from build123d import *

# Parameters (mm, degrees)
SKETCH_1_R          = 1.6
EXTRUDE_1_DEPTH     = 7
SKETCH_2_W          = 90
SKETCH_2_H          = 120
SKETCH_2_W_2        = 80
SKETCH_2_H_2        = 110
EXTRUDE_2_DEPTH     = 60
SKETCH_3_W          = 56
SKETCH_3_H          = 36
SKETCH_3_W_2        = 50
SKETCH_3_H_2        = 30
EXTRUDE_3_DEPTH     = 10
SKETCH_5_W          = 56
SKETCH_5_H          = 3
EXTRUDE_4_DEPTH     = 20
SKETCH_6_W          = 30
SKETCH_6_H          = 5
EXTRUDE_5_DEPTH     = 60
CUT_EXTRUDE_1_DEPTH = 10
EXTRUDE_6_DEPTH     = 5
CUT_EXTRUDE_2_DEPTH = 10
CUT_EXTRUDE_3_DEPTH = 10
CUT_EXTRUDE_4_DEPTH = 10


with BuildPart() as part:
    # 草图1 → 凸台-拉伸1 (new body)
    with BuildSketch(Plane(origin=(0, 0, 0), x_dir=(1, 0, 0), z_dir=(0, 1, 0))):
        with BuildLine():
            Line((-85.25974026, 139.090909091), (74.74025974, 139.090909091))
            ThreePointArc((74.74025974, 139.090909091), (81.811327552, 136.161976903), (84.74025974, 129.090909091))
            Line((84.74025974, 129.090909091), (84.74025974, -70.909090909))
            ThreePointArc((84.74025974, -70.909090909), (81.811327552, -77.980158721), (74.74025974, -80.909090909))
            Line((74.74025974, -80.909090909), (-85.25974026, -80.909090909))
            ThreePointArc((-85.25974026, -80.909090909), (-92.330808072, -77.980158721), (-95.25974026, -70.909090909))
            Line((-95.25974026, -70.909090909), (-95.25974026, 129.090909091))
            ThreePointArc((-95.25974026, 129.090909091), (-92.330808072, 136.161976903), (-85.25974026, 139.090909091))
        make_face()
        with Locations((-62.25974026, 89.090909091)):
            Circle(SKETCH_1_R, mode=Mode.SUBTRACT)
        with Locations((51.74025974, 89.090909091)):
            Circle(SKETCH_1_R, mode=Mode.SUBTRACT)
        with Locations((-62.25974026, -30.909090909)):
            Circle(SKETCH_1_R, mode=Mode.SUBTRACT)
        with Locations((51.74025974, -30.909090909)):
            Circle(SKETCH_1_R, mode=Mode.SUBTRACT)
    extrude(amount=EXTRUDE_1_DEPTH)

    # 草图2 → 凸台-拉伸2 (add)
    with BuildSketch(Plane.XZ):
        with Locations((-5.25974026, -64.090909091)):
            Rectangle(SKETCH_2_W, SKETCH_2_H)
        with Locations((-5.25974026, -64.090909091)):
            Rectangle(SKETCH_2_W_2, SKETCH_2_H_2, mode=Mode.SUBTRACT)
    extrude(amount=EXTRUDE_2_DEPTH)

    # 草图3 → 凸台-拉伸3 (add)
    with BuildSketch(Plane.XZ):
        with Locations((-5.25974026, 22.137368895)):
            Rectangle(SKETCH_3_W, SKETCH_3_H)
        with Locations((-5.25974026, 22.137368895)):
            Rectangle(SKETCH_3_W_2, SKETCH_3_H_2, mode=Mode.SUBTRACT)
    extrude(amount=EXTRUDE_3_DEPTH)

    # 草图5 → 凸台-拉伸4 (add)
    with BuildSketch(Plane.XZ.offset(10)):
        with Locations((-5.25974026, 5.637368895)):
            Rectangle(SKETCH_5_W, SKETCH_5_H)
    extrude(amount=EXTRUDE_4_DEPTH)

    # 草图6 → 凸台-拉伸5 (add)
    with BuildSketch(Plane.XZ):
        with Locations((-5.25974026, 69.33277689)):
            Rectangle(SKETCH_6_W, SKETCH_6_H)
    extrude(amount=EXTRUDE_5_DEPTH)

    # 草图8 → 切除-拉伸1 (cut)
    with BuildSketch(Plane.XY.offset(71.83277689)):
        with BuildLine():
            Line((-6.25974026, -43), (-10.25974026, -60))
            Line((-10.25974026, -60), (-0.25974026, -60))
            Line((-0.25974026, -60), (-4.25974026, -43))
            ThreePointArc((-4.25974026, -43), (-4.523672282, -41.881966011), (-5.25974026, -41))
            ThreePointArc((-5.25974026, -41), (-5.995808237, -41.881966011), (-6.25974026, -43))
        make_face()
    extrude(amount=-CUT_EXTRUDE_1_DEPTH, mode=Mode.SUBTRACT)

    # 草图9 → 凸台-拉伸6 (add)
    with BuildSketch(Plane.XY.offset(71.83277689)):
        Polygon((-6.25974026, -60), (-9.789152024, -58), (-10.25974026, -60), align=None)
        Polygon((-4.25974026, -60), (-0.25974026, -60), (-0.730328495, -58), align=None)
    extrude(amount=-EXTRUDE_6_DEPTH)

    # 草图10 → 切除-拉伸2 (cut)
    with BuildSketch(Plane.XZ):
        with BuildLine():
            Line((-64.659020205, -16.259764427), (-64.659020205, -61.488758584))
            ThreePointArc((-64.659020205, -61.488758584), (-73.36978945, -70.199527829), (-82.080558695, -61.488758584))
            Line((-82.080558695, -61.488758584), (-82.080558695, -16.259764427))
            ThreePointArc((-82.080558695, -16.259764427), (-73.36978945, -7.548995182), (-64.659020205, -16.259764427))
        make_face()
        with BuildLine():
            Line((67.459227113, -16.259764427), (67.459227113, -61.488758584))
            ThreePointArc((67.459227113, -61.488758584), (57.906863547, -71.04112215), (48.354499981, -61.488758584))
            Line((48.354499981, -61.488758584), (48.354499981, -16.259764427))
            ThreePointArc((48.354499981, -16.259764427), (57.906863547, -6.707400861), (67.459227113, -16.259764427))
        make_face()
    extrude(amount=-CUT_EXTRUDE_2_DEPTH, mode=Mode.SUBTRACT)

    # 草图11 → 切除-拉伸3 (cut)
    with BuildSketch(Plane.XZ):
        with BuildLine():
            Line((-80.892767317, 71.523985845), (-45.044601578, 71.523985845))
            ThreePointArc((-45.044601578, 71.523985845), (-38.176495058, 64.655879325), (-45.044601578, 57.787772805))
            Line((-45.044601578, 57.787772805), (-80.892767317, 57.787772805))
            ThreePointArc((-80.892767317, 57.787772805), (-87.760873837, 64.655879325), (-80.892767317, 71.523985845))
        make_face()
        with BuildLine():
            Line((39.550368976, 72.361559811), (65.180132332, 72.361559811))
            ThreePointArc((65.180132332, 72.361559811), (72.885812818, 64.655879325), (65.180132332, 56.950198839))
            Line((65.180132332, 56.950198839), (39.550368976, 56.950198839))
            ThreePointArc((39.550368976, 56.950198839), (31.84468849, 64.655879325), (39.550368976, 72.361559811))
        make_face()
    extrude(amount=-CUT_EXTRUDE_3_DEPTH, mode=Mode.SUBTRACT)

    # 草图12 → 切除-拉伸4 (cut)
    with BuildSketch(Plane.XZ):
        with BuildLine():
            Line((-65.903935016, -99.695986078), (-65.903935016, -125.770060152))
            ThreePointArc((-65.903935016, -125.770060152), (-72.642178878, -132.508304014), (-79.38042274, -125.770060152))
            Line((-79.38042274, -125.770060152), (-79.38042274, -99.695986078))
            ThreePointArc((-79.38042274, -99.695986078), (-72.642178878, -92.957742216), (-65.903935016, -99.695986078))
        make_face()
        with BuildLine():
            Line((66.517205225, -99.695986078), (66.517205225, -125.770060152))
            ThreePointArc((66.517205225, -125.770060152), (61.243796985, -131.043468392), (55.970388746, -125.770060152))
            Line((55.970388746, -125.770060152), (55.970388746, -99.695986078))
            ThreePointArc((55.970388746, -99.695986078), (61.243796985, -94.422577838), (66.517205225, -99.695986078))
        make_face()
    extrude(amount=-CUT_EXTRUDE_4_DEPTH, mode=Mode.SUBTRACT)


solid = part.part
Work out the finished part from the listing and answer in its coordinate system (mm). A direction names the side the tool comes from. Give positions to 0.01 mm unless a question says otherwise; leave off trailing zeros. Order: outer loops, then holes, each group sorted by start corner. A loop starts at its lowest first (then second) coordinate and runs counter-clockwise, first axis right, second up. Notation, with made-up numbers: (-7, 79.25) -> (32, 79.25) arc R28 cw to (32, 117.25) -> close; hole circle Ø8 at (44.5, 78.5). An arc over 180 degrees is marked (long way). Answer as a JSON object with one key per item and string values. Group by question number.
1. Section D-D on x = -14 is taken. Determine the outline of the cut face in (y, z), plus the area to 3 significant figures.
2. Section C-C on z = -49 is taken. Determine the outline of the cut face in (x, y).
3. Section B-B on y = -36 is taken. Determine the outline of the cut face in (x, z), plus the area to 3 significant figures.
4. A tool of negligible diameter and unlimited length cuts with its end or side. For faces 1 (the flat face through (-5, 0, 22)), 2 (the flat face through (-5, -30, 71.833)), 3 (the flat face through (-63, 3, 71.524)), from which of +Z, -Z, +X, -X, +Y, -Y can it reach the whole face along a straight path? Write none if from no direction.
5. Flat-ended cylindrical pins translate along their axes: pin 1 Ø18 at (x, y) = (-9.5, -28.5) entering from -Z; pin 2 Ø8 at (y, z) = (-5.5, 20) entering from +X; pin 3 Ø2 at (y, z) = (-37.5, -63) entering from +X. Find the tip coordinate at first contact, or state that the pin passes through.
6. The mould has two halves that part along X. Classify faces 4 (the cylindrical face through (-72.494, 3.451, -132.507)), 5 (the flat face through (39.74, -30, -65)), 6 (the flat face through (-5, -30, 66.833)), 7 (the flat face through (-95.26, 3, -28)): released by +X, released by -X, zero draft, split by the parting line, or undercut.
7. Section A-A on y = -23 is taken. Determine the outline of the cut face in (x, z).
8. Consider line 1 along Z through (x, y) = (-30.5, -14); line 2 along X through (y, z) = (-53, -20); line 3 along Z through (x, y) = (14.5, -3). Determine where each line is inside the solid, lowest interval first. Write a range as [from, to].
Result sheet:
{
 "1": {"outline": "(-60, -124.09) -> (0, -124.09) -> (0, -139.09) -> (7, -139.09) -> (7, 80.91) -> (0, 80.91) -> (0, 71.83) -> (-60, 71.83) -> (-60, 66.83) -> (0, 66.83) -> (0, 40.14) -> (-10, 40.14) -> (-10, 37.14) -> (0, 37.14) -> (0, 7.14) -> (-30, 7.14) -> (-30, 4.14) -> (0, 4.14) -> (0, -4.09) -> (-60, -4.09) -> (-60, -9.09) -> (0, -9.09) -> (0, -119.09) -> (-60, -119.09) -> close", "area": "2,560 mm^2"},
 "2": {"outline": "(-95.26, 0) -> (-82.08, 0) -> (-82.08, 7) -> (-95.26, 7) -> close; (-64.66, 0) -> (-50.26, 0) -> (-50.26, -60) -> (-45.26, -60) -> (-45.26, 0) -> (34.74, 0) -> (34.74, -60) -> (39.74, -60) -> (39.74, 0) -> (48.35, 0) -> (48.35, 7) -> (-64.66, 7) -> close; (67.46, 0) -> (84.74, 0) -> (84.74, 7) -> (67.46, 7) -> close"},
 "3": {"outline": "(-50.26, -124.09) -> (39.74, -124.09) -> (39.74, -4.09) -> (-50.26, -4.09) -> close; (-20.26, 66.83) -> (9.74, 66.83) -> (9.74, 71.83) -> (-20.26, 71.83) -> close; hole (-45.26, -119.09) -> (34.74, -119.09) -> (34.74, -9.09) -> (-45.26, -9.09) -> close", "area": "2,150 mm^2"},
 "4": {"face 1": "-Y", "face 2": "+Z, +X, -X, -Y", "face 3": "+Y, -Y"},
 "5": {"pin 1": "stops at z = -124.09", "pin 2": "stops at x = 22.74", "pin 3": "stops at x = 39.74"},
 "6": {"face 4": "undercut", "face 5": "released by +X", "face 6": "zero draft", "face 7": "released by -X"},
 "7": {"outline": "(-50.26, -124.09) -> (39.74, -124.09) -> (39.74, -4.09) -> (-50.26, -4.09) -> close; (-33.26, 4.14) -> (22.74, 4.14) -> (22.74, 7.14) -> (-33.26, 7.14) -> close; (-20.26, 66.83) -> (9.74, 66.83) -> (9.74, 71.83) -> (-20.26, 71.83) -> close; hole (-45.26, -119.09) -> (34.74, -119.09) -> (34.74, -9.09) -> (-45.26, -9.09) -> close"},
 "8": {"line 1": "z = [-124.09, -119.09], [-9.09, -4.09], [4.14, 7.14]", "line 2": "x = [-50.26, -45.26], [34.74, 39.74]", "line 3": "z = [-124.09, -119.09], [-9.09, -4.09], [4.14, 7.14], [37.14, 40.14]"}
}
